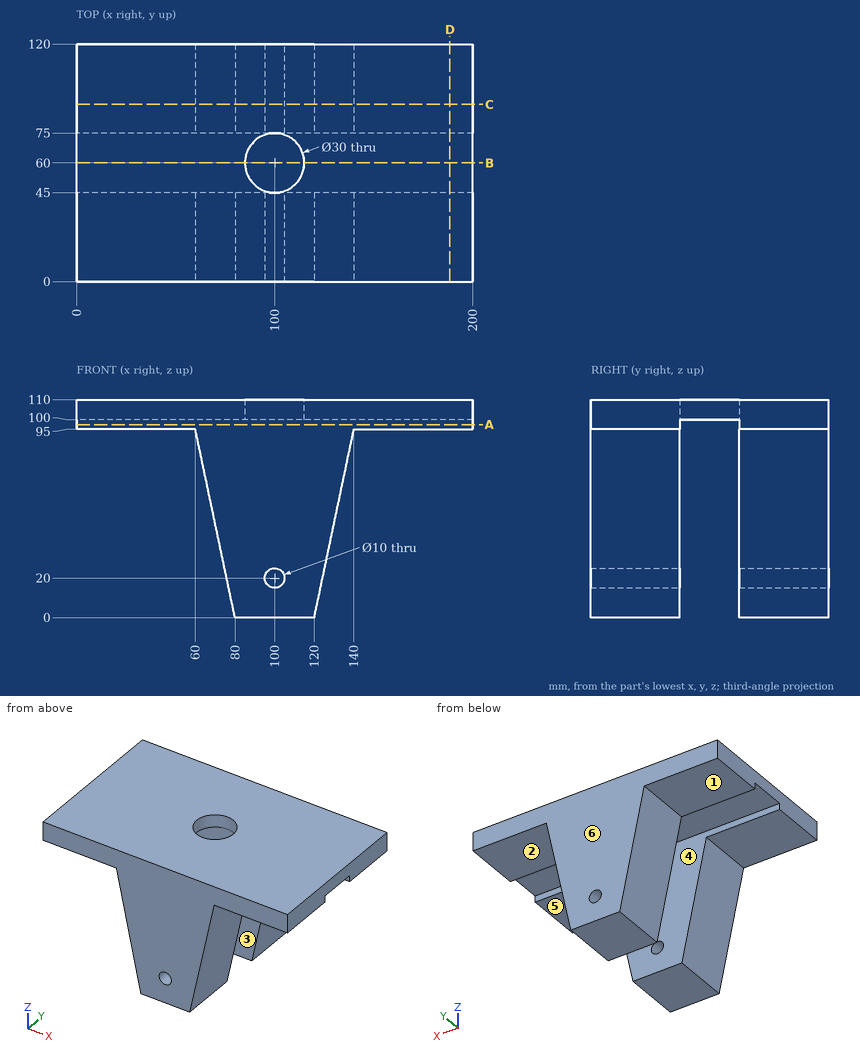
Study the drawing (mm; zero at the part's minimum x, y, z) and answer. A direction names the side the tool comes from. Give positions to 0.01 mm unless a question says otherwise; leave off trailing zeros. Loops run counter-clockwise (first coordinate to the right, second up) from the corner with the lowest first, then second, coordinate; pieces in that order, holes last. Notation, with made-up numbers: (44.25, -35.75) - (91.25, -35.75) arc R31 cw to (91.25, -5.75) - close; hole circle Ø2 at (4, 12). An arc over 180 degrees is marked (long way). Return JSON: item names as keys, results as strings. Group by question number.
1. Which of the six approach directions +Z, -Z, +X, -X, +Y, -Y give full straight-line access (tool end or side, diameter ignored) to the marked faces 1, 2 and 3?
2. Find section D-D (x = 188.5). Write down the section's boundary in (y, z).
3. Given pin 1 Ø5 at (x, y) = (93, 13) entering from -Z; pin 2 Ø8 at (x, z) = (100, 20) entering from +Y; pin 3 Ø1 at (y, z) = (25.5, 12) entering from -X; pin 4 Ø24 at (x, y) = (48.5, 55.5) entering from -Z, each flat-ended and moving along its own axis, determine where each tip first touches the part or whether it passes through.
4. Straight lines are drawn through the part: line 1 (Y direction, x = 167.5, z = 97.5); line 2 (Z direction, x = 100, y = 89.5); line 3 (Z direction, x = 21.5, y = 45.5). For each, find the intervals that lie inside material, in ascending order. Write a range as [from, to].
5. Find section C-C (y = 89.5). Write down the section's boundary in (x, z), then the cut area to 3 significant figures.
6. Find section B-B (y = 60). Write down the section's boundary in (x, z).
7. Find section A-A (z = 97.5). Write down the section's boundary in (x, y), then the cut area to 3 significant figures.
8. Determine the mould class of the marked faces 4, 5 and 6 for opening direction Y: pulls with the +Y half, pulls with the -Y half, needs draft (parallel to the pull), parting line crosses it, or undercut.
Verdict:
{
 "1": {"face 1": "-Z, -X, +Y, -Y", "face 2": "-Z, +X, +Y, -Y", "face 3": "-Z, +X, -X"},
 "2": {"outline": "(0, 95) - (45, 95) - (45, 100) - (75, 100) - (75, 95) - (120, 95) - (120, 110) - (0, 110) - close"},
 "3": {"pin 1": "stops at z = 0", "pin 2": "passes through", "pin 3": "stops at x = 77.37", "pin 4": "stops at z = 95"},
 "4": {"line 1": "y = [0, 45], [75, 120]", "line 2": "z = [0, 15], [25, 110]", "line 3": "z = [100, 110]"},
 "5": {"outline": "(0, 95) - (60, 95) - (80, 0) - (120, 0) - (140, 95) - (200, 95) - (200, 110) - (0, 110) - close; hole circle Ø10 at (100, 20)", "area": "8,620 mm^2"},
 "6": {"outline": "(0, 100) - (85, 100) - (85, 110) - (0, 110) - close; (115, 100) - (200, 100) - (200, 110) - (115, 110) - close"},
 "7": {"outline": "(0, 0) - (200, 0) - (200, 45) - (0, 45) - close; (0, 75) - (200, 75) - (200, 120) - (0, 120) - close", "area": "18,000 mm^2"},
 "8": {"face 4": "undercut", "face 5": "needs draft", "face 6": "pulls with the +Y half"}
}
